```python
from build123d import *

# Parameters (mm, degrees)
F0_R     = 4.5
F0_R_2   = 2.5
F1_DEPTH = 35
F2_DEPTH = 27
F3_SIZE  = 0.8
F4_SIZE  = 0.5


with BuildPart() as f1:
    # F0 (on Front) → F1 (new body, symmetric)
    with BuildSketch(Plane.XZ):
        Circle(F0_R)
        Circle(F0_R_2, mode=Mode.SUBTRACT)
        Circle(F0_R_2)
    extrude(amount=F1_DEPTH, both=True)

    # F0 (on Front) → F2 (cut, symmetric)
    with BuildSketch(Plane.XZ):
        Circle(F0_R)
        Circle(F0_R_2, mode=Mode.SUBTRACT)
    extrude(amount=F2_DEPTH, both=True, mode=Mode.SUBTRACT)

    # F3
    f3_edges = [f1.edges().sort_by_distance(p)[0] for p in [
        (-4.5, 35, 0),
        (-4.5, -35, 0),
    ]]
    chamfer(f3_edges, length=F3_SIZE)

    # F4
    f4_edges = [f1.edges().sort_by_distance(p)[0] for p in [
        (-4.5, 27, 0),
        (-4.5, -27, 0),
    ]]
    chamfer(f4_edges, length=F4_SIZE)


solid = f1.part
```
The listing builds one solid part. Answer for the finished solid, in the listing's coordinates (mm). A direction names the side the tool comes from. Round coordinates to 2 decimals unless told otherwise and drop trailing zeros. Order: outer loops, then holes, each group sorted by start corner. A loop starts at its lowest first (then second) coordinate and runs counter-clockwise, first axis right, second up. Notation, with made-up numbers: (5, -20) -> (24, -20) arc R19 cw to (24, -2) -> close; hole circle Ø8 at (49.25, 4.25). An arc over 180 degrees is marked (long way). Answer as CSV lines item,"result". Start each with the question number.
(1) For a pull along Y with two mould halves and no side action, classify faces 3 (the face through (0, 35, 0)), 4 (the face through (-2, 27, -2)), 5 (the face through (0, -35, 0)) as +Y half, -Y half, draft (parallel to the pull), parting line (faces both ways), or undercut.
(2) Find the intervals of material crossed by probe 1 along Y at (x, z) = (-1.5, -2.75); probe 2 along Y at (x, z) = (-2.25, 3); probe 3 along X at (y, z) = (20, 0.75), in increasing order. Write a range as from..to.
(3) The part is cut by section C-C (y = -12). Determine the outline of the cut face in (x, z), then the cut area to 3 significant figures.
(4) The part is cut by section B-B (z = 0). Determine the outline of the cut face in (x, y), then the cut area to 3 significant figures.
(5) A tool of negligible diameter and unlimited length cuts with its end or side. For faces 1 (the face through (-0.59, 30.8, 4.46)), 2 (the face through (-0.54, 0.38, -2.44)), from which of +Z, -Z, +X, -X, +Y, -Y can it reach the whole face along a straight path? Write none if from no direction.
(6) Flat-ended cylindrical pins translate along their axes: pin 1 Ø1 at (x, y) = (0.5, -16) entering from +Z; pin 2 Ø2 at (x, y) = (2.5, 24.5) entering from +Z; pin 3 Ø4 at (x, y) = (-2.5, -4.5) entering from -Z. Find the tip coordinate at first contact, or state that the pin passes through.
(7) The part is cut by section A-A (x = 0). Determine the outline of the cut face in (y, z).
Evaluation:
1,face 3,"+Y half"
1,face 4,"undercut"
1,face 5,"-Y half"
2,probe 1,"-35..-27, 27..35"
2,probe 2,"-34.95..-27, 27..34.95"
2,probe 3,"-2.38..2.38"
3,outline,"circle Ø5 at (0, 0)"
3,area,"19.6 mm²"
4,outline,"(-4.5, -34.2) -> (-3.7, -35) -> (3.7, -35) -> (4.5, -34.2) -> (4.5, -27.5) -> (4, -27) -> (2.5, -27) -> (2.5, 27) -> (4, 27) -> (4.5, 27.5) -> (4.5, 34.2) -> (3.7, 35) -> (-3.7, 35) -> (-4.5, 34.2) -> (-4.5, 27.5) -> (-4, 27) -> (-2.5, 27) -> (-2.5, -27) -> (-4, -27) -> (-4.5, -27.5) -> close"
4,area,"412 mm²"
5,face 1,"+Y, -Y"
5,face 2,"none"
6,pin 1,"z = 2.5"
6,pin 2,"z = 2"
6,pin 3,"z = -2.45"
7,outline,"(-35, -3.7) -> (-34.2, -4.5) -> (-27.5, -4.5) -> (-27, -4) -> (-27, -2.5) -> (27, -2.5) -> (27, -4) -> (27.5, -4.5) -> (34.2, -4.5) -> (35, -3.7) -> (35, 3.7) -> (34.2, 4.5) -> (27.5, 4.5) -> (27, 4) -> (27, 2.5) -> (-27, 2.5) -> (-27, 4) -> (-27.5, 4.5) -> (-34.2, 4.5) -> (-35, 3.7) -> close"
